```python
from build123d import *

# Parameters (mm, degrees)
SKETCH2_R               = 1
CUT_EXTRUDE1_DEPTH      = 7
CUT_EXTRUDE1_DEPTH_BACK = 7
SKETCH3_W               = 2
SKETCH3_H               = 1
SKETCH4_R               = 4
CUT_EXTRUDE2_DEPTH      = 2
SKETCH5_R               = 3
BOSS_EXTRUDE1_DEPTH     = 32.4


with BuildPart() as part:
    # Sketch1 → Revolve1 (revolve)
    with BuildSketch(Plane.XY):
        with BuildLine():
            Line((0, 4), (34.4, 4))
            Line((34.4, 4), (34.4, 6))
            ThreePointArc((34.4, 6), (37.030951895, 3.498571137), (38, 0))
            Line((38, 0), (0, 0))
            Line((0, 0), (0, 4))
        make_face()
    revolve(axis=Axis((0, 0, 0), (1, 0, 0)))

    # Sketch2 → Cut-Extrude1 (cut, two sides)
    with BuildSketch(Plane(origin=(0, 0, 0), x_dir=(1, 0, 0), z_dir=(0, 1, 0))) as cut_extrude1_sk:
        with Locations((4.6, 0)):
            Circle(SKETCH2_R)
    extrude(amount=CUT_EXTRUDE1_DEPTH, mode=Mode.SUBTRACT)
    extrude(cut_extrude1_sk.sketch, amount=-CUT_EXTRUDE1_DEPTH_BACK, mode=Mode.SUBTRACT)

    # Sketch3 → Cut-Revolve1 (revolve, cut)
    with BuildSketch(Plane(origin=(0, 0, 0), x_dir=(1, 0, 0), z_dir=(0, 1, 0))):
        with Locations((4.6, 3.5)):
            Rectangle(SKETCH3_W, SKETCH3_H)
    revolve(axis=Axis((34.4, 0, 0), (-1, 0, 0)), mode=Mode.SUBTRACT)

    # Sketch4 → Cut-Extrude2 (cut)
    with BuildSketch(Plane.ZY):
        Circle(SKETCH4_R)
    extrude(amount=-CUT_EXTRUDE2_DEPTH, mode=Mode.SUBTRACT)

    # Sketch5 → Boss-Extrude1 (add)
    with BuildSketch(Plane.ZY.offset(-2)):
        Circle(SKETCH5_R)
    extrude(amount=-BOSS_EXTRUDE1_DEPTH)


solid = part.part
```
Check sheet for the modelled part. Datum: model origin and axes. Units: mm. A direction names the side the tool comes from. Coordinates: 2 decimals unless noted, no trailing zeros. Write each loop counter-clockwise with the first axis right and the second up, starting at its lowest first coordinate (ties: lowest second). Pieces come first, ordered by that corner, then holes. Notation, with made-up numbers: (-18.75, 78) - (5.25, 78) arc R10 ccw to (5.25, 90) - close; hole circle Ø3 at (17.25, 26.25). An arc over 180 degrees is marked (long way). One line per question, with ' | ' between items.
Item 1: Thickness scan on line 1 (X direction, y = -2.75, z = 1.75); line 2 (Y direction, x = 20.5, z = 0); line 3 (Z direction, x = 34.5, y = -1.25). Record the ranges inside material, lowest first. Write a range as [from, to].
Determined:
line 1: x = [2, 3.6], [5.6, 37.17] | line 2: y = [-4, 4] | line 3: z = [-5.81, 5.81]
Item 2: Sectioned sample at D-D on x = 31.5. Record the boundary of the cut face in (y, z), plus the area to 3 significant figures.
Determined:
outline: circle Ø8 at (0, 0) | area: 50.3 mm2
Item 3: Sectioned sample at C-C on z = -2.25. Record the boundary of the cut face in (x, y), plus the area to 3 significant figures.
Determined:
outline: (2, -3.31) - (3.6, -3.31) - (3.6, -1.98) - (5.6, -1.98) - (5.6, -3.31) - (34.4, -3.31) - (34.4, -5.56) arc R6.42 ccw to (34.4, 5.56) - (34.4, 3.31) - (5.6, 3.31) - (5.6, 1.98) - (3.6, 1.98) - (3.6, 3.31) - (2, 3.31) - close | area: 234 mm2
Item 4: Gauge pin test, flat ends, axial feed: P1, Ø4, axis at y = 1.5, z = 1.5, coming from the +X side; P2, Ø6, axis at x = 6.5, z = 0.5, coming from the -Y side; P3, Ø1, axis at y = 4, z = 1, coming from the +X side. Record the tip position at first contact, or that the pin passes through.
Determined:
P1: stops at x = 38 | P2: stops at y = -4 | P3: stops at x = 36.95
Item 5: Sectioned sample at B-B on y = 0. Record the boundary of the cut face in (x, z), plus the area to 3 significant figures.
Determined:
outline: (2, -4) - (3.6, -4) - (3.6, -3) - (5.6, -3) - (5.6, -4) - (34.4, -4) - (34.4, -6) arc R6.8 ccw to (34.4, 6) - (34.4, 4) - (5.6, 4) - (5.6, 3) - (3.6, 3) - (3.6, 4) - (2, 4) - close | area: 286 mm2
Item 6: Mould release check, pull along X, two halves, no side actions. Record for faces 1 (the face through (34.4, 1.42, -3.92)), 2 (the face through (5.6, -3, 1)), 3 (the face through (20.202, -0.867, -3.905)), 4 (the face through (3.6, -3, 1)): pulls with the +X half, pulls with the -X half, needs draft (parallel to the pull), parting line crosses it, or undercut.
Determined:
face 1: pulls with the -X half | face 2: undercut | face 3: needs draft | face 4: undercut
Item 7: Sectioned sample at A-A on z = 3.5. Record the boundary of the cut face in (x, y).
Determined:
outline: (2, -1.94) - (3.6, -1.94) - (3.6, 1.94) - (2, 1.94) - close; (5.6, -1.94) - (34.4, -1.94) - (34.4, -4.87) arc R5.83 ccw to (34.4, 4.87) - (34.4, 1.94) - (5.6, 1.94) - close
Item 8: Access from +Z, -Z, +X, -X, +Y, -Y to the whole of each face (thin tool, end or side, straight path). Record for faces 5 (the face through (2.811, 3.815, 1.201)), 6 (the face through (2, 0, 0)).
Determined:
face 5: -X | face 6: +Z, -Z, -X, +Y, -Y
